Model file for the job. Use its own axes, mm. Round coordinates to 2 decimals unless told otherwise and drop trailing zeros. Write each loop counter-clockwise with the first axis right and the second up, starting at its lowest first coordinate (ties: lowest second). Pieces come first, ordered by that corner, then holes. Notation, with made-up numbers: (73.5, 43.5) - (94.5, 43.5) arc R18 cw to (94.5, 58.5) - close; hole circle Ø4 at (-28, 85). An arc over 180 degrees is marked (long way). One line per item, written item: value.
from build123d import *

# Parameters (mm, degrees)
IZIM1_R                     = 6
IZIM1_R_2                   = 4
Y_KSEKLIK_EKSTR_ZYON1_DEPTH = 4.5
BOSS_EXTRUDE1_START         = 4
SKETCH1_R                   = 6
SKETCH1_R_2                 = 4
BOSS_EXTRUDE1_DEPTH         = 4


with BuildPart() as part:
    # Çizim1 → Yükseklik-Ekstrüzyon1 (new body)
    with BuildSketch(Plane(origin=(0, 0, 0), x_dir=(1, 0, 0), z_dir=(0, 1, 0))):
        with Locations(Location((0, 0, 0), (0, 0, 270))):
            Circle(IZIM1_R)
        with Locations(Location((0, 0, 0), (0, 0, 270))):
            Circle(IZIM1_R_2, mode=Mode.SUBTRACT)
    extrude(amount=Y_KSEKLIK_EKSTR_ZYON1_DEPTH)

    # Çizim2 → Döndür1 (revolve)
    with BuildSketch(Plane(origin=(0, 0, 0), x_dir=(0, 0, -1), z_dir=(1, 0, 0))):
        with BuildLine():
            Line((0, 4.5), (0, 6.005722605))
            ThreePointArc((0, 6.005722605), (3.083863381, 5.587039913), (6, 4.5))
            Line((6, 4.5), (0, 4.5))
        make_face()
    revolve(axis=Axis((0, 4.5, 0), (0, 1, 0)))

    # Sketch1 → Boss-Extrude1 (add)
    with BuildSketch(Plane.XZ.offset(BOSS_EXTRUDE1_START)):
        with Locations(Location((0, 0, 0), (0, 0, 270))):
            Circle(SKETCH1_R)
        with Locations(Location((0, 0, 0), (0, 0, 270))):
            Circle(SKETCH1_R_2, mode=Mode.SUBTRACT)
    extrude(amount=-BOSS_EXTRUDE1_DEPTH)


solid = part.part
1. Band-saw the part on A-A on y = 2. Write the cut outline in (x, z).
Report:
outline: circle Ø12 at (0, 0); hole circle Ø8 at (0, 0)
2. Mould opens along Z. For faces 1 (the face through (0, 4.5, 0)), 2 (the face through (-3.92, -4, 1.42)) say: released by +Z, released by -Z, zero draft, split by the parting line, or undercut.
Report:
face 1: undercut
face 2: zero draft
3. Wall check: probe 1 along Z at (x, y) = (0, -1); probe 2 along Z at (x, y) = (3, 3.25). Give the ranges that are in metal, low to high. Write a range as [from, to].
Report:
probe 1: [-6, -4], [4, 6]
probe 2: [-5.2, -2.65], [2.65, 5.2]
4. Drop flat-ended pins along their axis: pin 1 (2.5 mm diameter, centred on x = -0.5, z = -0.5, fed in from -Y); pin 2 (1.5 mm diameter, centred on y = -2.5, z = 4, fed in from +X); pin 3 (1.5 mm diameter, centred on y = 1.5, z = -2, fed in from -X). Give the stop position or say it passes through.
Report:
pin 1: y = 4.5
pin 2: x = 5.04
pin 3: x = -5.87
